Geometry check sheet. Reference: the model listing, model coordinates, mm. Face numbers are marked on the shaded views. A direction names the side the tool comes from. Give positions to 0.01 mm unless a question says otherwise; leave off trailing zeros. Loops run counter-clockwise (first coordinate to the right, second up) from the corner with the lowest first, then second, coordinate; pieces in that order, holes last.
1. Cross-section at B-B, the plane y = 15.25. Record the cut outline in (x, z), plus the area to 3 significant figures.
2. Cross-section at A-A, the plane z = 0. Record the cut outline in (x, y).
3. Go/stop test with flat-tipped pins: pin 1 Ø6 at (y, z) = (10.5, 3.5) entering from -X; pin 2 Ø4 at (x, z) = (-6.5, 0) entering from +Y; pin 3 Ø1.2 at (x, y) = (-15, 17.5) entering from -Z; pin 4 Ø3 at (x, z) = (6.5, 0) entering from +Y. Record where each tip stops, or that it passes through.
4. Material ranges on L1, parallel to X at y = 17.1, z = 0; L2, parallel to X at y = 2.1, z = 0; L3, parallel to Z at x = -6.5, y = 9.75, recorded low to high.
5. Cross-section at C-C, the plane x = -14. Record the cut outline in (y, z), plus the area to 3 significant figures.
6. Cross-section at D-D, the plane y = 9.5. Record the cut outline in (x, z).
7. Release check for a two-part mould opening along X. For the marked faces 1, 2, 3 and 4 record: +X half, -X half, draft (parallel to the pull), parting line (faces both ways), or undercut.
8. Tool access check on the marked faces 5, 6 and 7. Record the directions out of +Z, -Z, +X, -X, +Y, -Y that give a thin tool (end or side, any length) a straight path to the whole face; none if there is none.
from build123d import *

# Parameters (mm, degrees)
SKETCH1_W               = 20
SKETCH1_H               = 20
BOSS_EXTRUDE1_DEPTH     = 20
SKETCH2_R               = 4.25
CUT_EXTRUDE1_DEPTH      = 10
SKETCH3_R               = 1.75
CUT_EXTRUDE2_DEPTH      = 25.494897428
SKETCH4_R               = 3
CUT_EXTRUDE3_DEPTH      = 15
SKETCH5_W               = 8
SKETCH5_H               = 4
BOSS_EXTRUDE2_DEPTH     = 8
CUT_EXTRUDE4_DEPTH      = 27.076809621
CUT_EXTRUDE4_DEPTH_BACK = 27.076809621
SKETCH6_R               = 1.75


with BuildPart() as part:
    # Sketch1 → Boss-Extrude1 (new body)
    with BuildSketch(Plane(origin=(0, 0, 0), x_dir=(1, 0, 0), z_dir=(0, 1, 0))):
        Rectangle(SKETCH1_W, SKETCH1_H)
    extrude(amount=BOSS_EXTRUDE1_DEPTH)

    # Sketch2 → Cut-Extrude1 (cut)
    with BuildSketch(Plane(origin=(0, 20, 0), x_dir=(1, 0, 0), z_dir=(0, 1, 0))):
        with Locations(Location((0, 0, 0), (0, 0, 270))):
            Circle(SKETCH2_R)
    extrude(amount=-CUT_EXTRUDE1_DEPTH, mode=Mode.SUBTRACT)

    # Sketch3 → Cut-Extrude2 (cut, through all)
    with BuildSketch(Plane(origin=(0, 20, 0), x_dir=(1, 0, 0), z_dir=(0, 1, 0))):
        with Locations(Location((-6.5, 0, 0), (0, 0, 270))):
            Circle(SKETCH3_R)
        with Locations(Location((6.5, 0, 0), (0, 0, 270))):
            Circle(SKETCH3_R)
    extrude(amount=-CUT_EXTRUDE2_DEPTH, mode=Mode.SUBTRACT)

    # Sketch4 → Cut-Extrude3 (cut)
    with BuildSketch(Plane(origin=(0, 20, 0), x_dir=(1, 0, 0), z_dir=(0, 1, 0))):
        with Locations(Location((-6.5, 0, 0), (0, 0, 270))):
            Circle(SKETCH4_R)
        with Locations(Location((6.5, 0, 0), (0, 0, 270))):
            Circle(SKETCH4_R)
    extrude(amount=-CUT_EXTRUDE3_DEPTH, mode=Mode.SUBTRACT)

    # Sketch5 → Boss-Extrude2 (add)
    with BuildSketch(Plane.ZY.offset(10)):
        with Locations((0, 18)):
            Rectangle(SKETCH5_W, SKETCH5_H)
    extrude(amount=BOSS_EXTRUDE2_DEPTH)

    # Sketch6 → Cut-Extrude4 (cut, two sides: drawn at the far end of the back side and taken through both)
    with BuildSketch(Plane.XZ.offset(-16).offset(-CUT_EXTRUDE4_DEPTH_BACK)):
        with Locations(Location((-14, 0, 0), (0, 0, 270))):
            Circle(SKETCH6_R)
    extrude(amount=CUT_EXTRUDE4_DEPTH + CUT_EXTRUDE4_DEPTH_BACK, mode=Mode.SUBTRACT)


solid = part.part
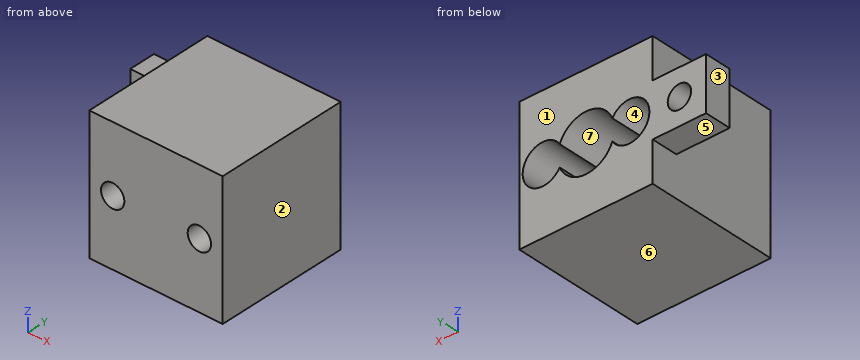
Result:
1. outline: (-10, -10) - (10, -10) - (10, 10) - (-10, 10) - close; hole (-3.95, -1.58) arc R4.25 ccw to (3.95, -1.58) arc R3 ccw (long way) to (3.95, 1.58) arc R4.25 ccw to (-3.95, 1.58) arc R3 ccw (long way) to start
1. area: 290 mm2
2. outline: (-18, 16) - (-15.75, 16) - (-15.75, 20) - (-18, 20) - close; (-12.25, 16) - (-10, 16) - (-10, 0) - (-8.25, 0) - (-8.25, 5) - (-9.5, 5) - (-9.5, 20) - (-12.25, 20) - close; (-4.75, 0) - (4.75, 0) - (4.75, 5) - (3.5, 5) - (3.5, 10) - (-3.5, 10) - (-3.5, 5) - (-4.75, 5) - close; (8.25, 0) - (10, 0) - (10, 20) - (9.5, 20) - (9.5, 5) - (8.25, 5) - close
3. pin 1: stops at x = -10
3. pin 2: stops at y = 5
3. pin 3: stops at z = -4
3. pin 4: passes through
4. L1: x = -18 to -15.75, -12.25 to -9.5, 9.5 to 10
4. L2: x = -10 to -8.25, -4.75 to 4.75, 8.25 to 10
4. L3: z = -10 to -3, 3 to 10
5. outline: (16, -4) - (20, -4) - (20, -1.75) - (16, -1.75) - close; (16, 1.75) - (20, 1.75) - (20, 4) - (16, 4) - close
5. area: 18.0 mm2
6. outline: (-10, -10) - (10, -10) - (10, 10) - (-10, 10) - close; hole circle Ø6 at (-6.5, 0); hole circle Ø6 at (6.5, 0)
7. face 1: draft
7. face 2: +X half
7. face 3: -X half
7. face 4: undercut
8. face 5: -Z, -X, +Y, -Y
8. face 6: -Z, +X, -X, +Y, -Y
8. face 7: +Y
